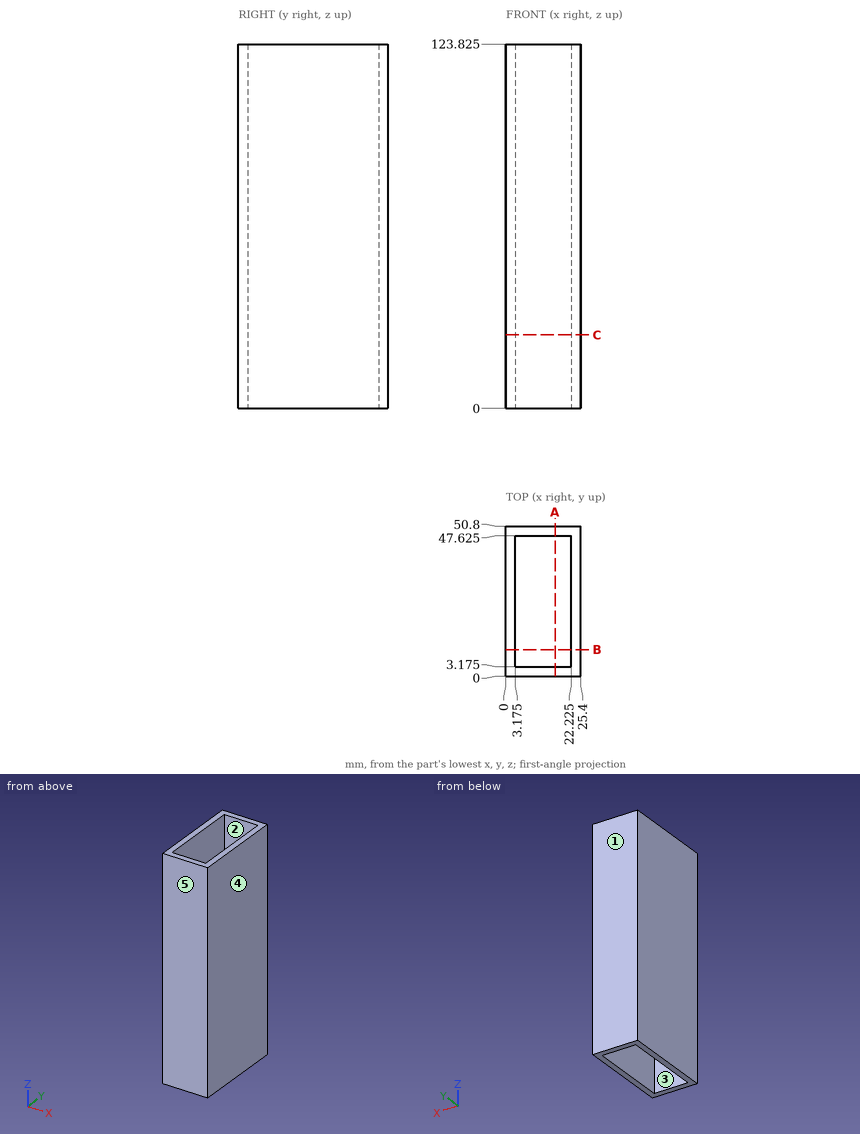
Geometry check sheet. Reference: drawing and pictorial views, mm from the part's lowest x, y, z. A direction names the side the tool comes from. Round coordinates to 2 decimals unless told otherwise and drop trailing zeros. Loops run counter-clockwise (first coordinate to the right, second up) from the corner with the lowest first, then second, coordinate; pieces in that order, holes last. Notation, with made-up numbers: (11.25, 18) - (69.25, 18) arc R19 cw to (69.25, 34) - close; hole circle Ø5 at (-19, -18.75). An arc over 180 degrees is marked (long way). Answer in a Markdown table with one row per item. Add a question column.
Q1. Section check C-C on z = 25. Enter the section's corners in (x, y) (3 decimals).
Q2. Section check B-B on y = 9. Enter the section's corners in (x, z) (3 decimals).
Q3. Material ranges on line 1 (Y direction, x = 6.75, z = 82) (3 decimals); line 2 (X direction, y = 8.5, z = 59.5) (3 decimals), recorded low to high.
Q4. Release check for a two-part mould opening along Y. For the marked faces 3, 4 and 5 record: pulls with the +Y half, pulls with the -Y half, needs draft (parallel to the pull), parting line crosses it, or undercut.
Q5. Tool access check on the marked faces 1 and 2. Record the directions out of +Z, -Z, +X, -X, +Y, -Y that give a thin tool (end or side, any length) a straight path to the whole face; none if there is none.
Q6. Section check A-A on x = 16.75. Enter the section's corners in (y, z) (3 decimals), plus the area to 3 significant figures.
Found:
| question | item | result |
|---|---|---|
| 1 | outline | (0, 0) - (25.4, 0) - (25.4, 50.8) - (0, 50.8) - close; hole (3.175, 3.175) - (22.225, 3.175) - (22.225, 47.625) - (3.175, 47.625) - close |
| 2 | outline | (0, 0) - (3.175, 0) - (3.175, 123.825) - (0, 123.825) - close; (22.225, 0) - (25.4, 0) - (25.4, 123.825) - (22.225, 123.825) - close |
| 3 | line 1 | y = 0 to 3.175, 47.625 to 50.8 |
| 3 | line 2 | x = 0 to 3.175, 22.225 to 25.4 |
| 4 | face 3 | undercut |
| 4 | face 4 | needs draft |
| 4 | face 5 | pulls with the -Y half |
| 5 | face 1 | +Z, -Z, +X, -X, +Y |
| 5 | face 2 | +Z, -Z |
| 6 | outline | (0, 0) - (3.175, 0) - (3.175, 123.825) - (0, 123.825) - close; (47.625, 0) - (50.8, 0) - (50.8, 123.825) - (47.625, 123.825) - close |
| 6 | area | 786 mm² |
